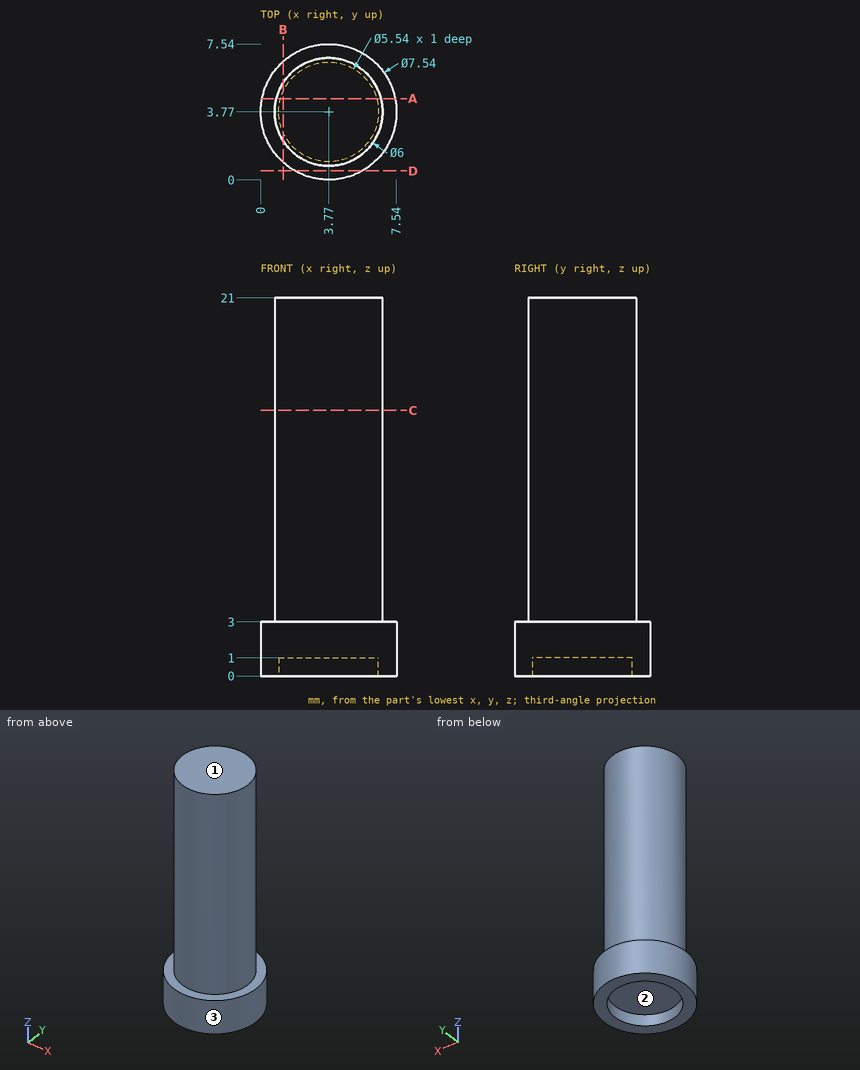
Geometry check sheet. Reference: drawing and pictorial views, mm from the part's lowest x, y, z. Round coordinates to 2 decimals unless told otherwise and drop trailing zeros. Loops run counter-clockwise (first coordinate to the right, second up) from the corner with the lowest first, then second, coordinate; pieces in that order, holes last. Notation, with made-up numbers: (71, 77) -> (115, 77) arc R26 ccw to (115, 112) -> close; hole circle Ø11 at (45.25, -25.5). An arc over 180 degrees is marked (long way). Answer as a JSON object with one key per item and string values.
Q1. Section check A-A (y = 4.5). Record the boundary of the cut face in (x, z), then the cut area to 3 significant figures.
Data:
{"outline": "(0.07, 0) -> (1.1, 0) -> (1.1, 1) -> (6.44, 1) -> (6.44, 0) -> (7.47, 0) -> (7.47, 3) -> (6.68, 3) -> (6.68, 21) -> (0.86, 21) -> (0.86, 3) -> (0.07, 3) -> close", "area": "122 mm2"}
Q2. Scan lines: line 1 (Z direction, x = 6.25, y = 6); line 2 (Z direction, x = 1.5, y = 3); line 3 (Y direction, x = 2, z = 4.75). Record each from-to range of solid material in increasing order. Write a range as from..to.
Data:
{"line 1": "z = 0..3", "line 2": "z = 1..21", "line 3": "y = 1.35..6.19"}
Q3. Section check C-C (z = 14.75). Record the boundary of the cut face in (x, y), then the cut area to 3 significant figures.
Data:
{"outline": "circle Ø6 at (3.77, 3.77)", "area": "28.3 mm2"}
Q4. Draft check along Y on the marked faces 1, 2 and 3. Enter one of: pulls with the +Y half, pulls with the -Y half, needs draft (parallel to the pull), parting line crosses it, or undercut.
Data:
{"face 1": "needs draft", "face 2": "undercut", "face 3": "parting line crosses it"}
Q5. Section check B-B (x = 1.25). Record the boundary of the cut face in (y, z), then the cut area to 3 significant figures.
Data:
{"outline": "(0.97, 0) -> (2.62, 0) -> (2.62, 1) -> (4.92, 1) -> (4.92, 0) -> (6.57, 0) -> (6.57, 3) -> (5.4, 3) -> (5.4, 21) -> (2.14, 21) -> (2.14, 3) -> (0.97, 3) -> close", "area": "73.1 mm2"}
Q6. Section check D-D (y = 0.5). Record the boundary of the cut face in (x, z), then the cut area to 3 significant figures.
Data:
{"outline": "(1.89, 0) -> (5.65, 0) -> (5.65, 3) -> (1.89, 3) -> close", "area": "11.3 mm2"}
Q7. Go/stop test with flat-tipped pins: P1, Ø1.5, axis at x = 5, z = 7.5, coming from the +Y side; P2, Ø4, axis at y = 1, z = 10.5, coming from the -X side; P3, Ø3, axis at x = 2, z = 18, coming from the +Y side. Record where each tip stops, or that it passes through.
Data:
{"P1": "stops at y = 6.73", "P2": "stops at x = 0.87", "P3": "stops at y = 6.76"}
